Work out the finished part from the listing and answer in its coordinate system (mm). A direction names the side the tool comes from. Coordinates: 2 decimals unless noted, no trailing zeros. Order: outer loops, then holes, each group sorted by start corner. A loop starts at its lowest first (then second) coordinate and runs counter-clockwise, first axis right, second up. Notation, with made-up numbers: (15.5, 33) -> (46.5, 33) arc R14 cw to (46.5, 50) -> close; hole circle Ø11 at (72, 55). An arc over 180 degrees is marked (long way). Use one line per item in the form item = value.
from build123d import *

# Parameters (mm, degrees)
SKETCH1_W                      = 119.888
SKETCH1_H                      = 182.88
BOSS_EXTRUDE1_DEPTH            = 9.525
F_1_4_20_TAPPED_HOLE1_D        = 5.1054
CUT_EXTRUDE1_DEPTH             = 1.9685
CUT_EXTRUDE2_DEPTH             = 1.9685
F_6_32_TAPPED_HOLE1_AT_2_COUNT = 2
F_6_32_TAPPED_HOLE1_AT_2_PITCH = 93.98
F_6_32_TAPPED_HOLE1_AT_3_COUNT = 2
F_6_32_TAPPED_HOLE1_AT_3_PITCH = 82.55
F_6_32_TAPPED_HOLE1_AT_4_COUNT = 2
F_6_32_TAPPED_HOLE1_AT_4_PITCH = 11.43


with BuildPart() as part:
    # Sketch1 → Boss-Extrude1 (new body)
    with BuildSketch(Plane(origin=(0, 0, 0), x_dir=(1, 0, 0), z_dir=(0, 1, 0))):
        Rectangle(SKETCH1_W, SKETCH1_H)
        with BuildLine():
            Line((-29.26715, 79.502), (29.26715, 79.502))
            ThreePointArc((29.26715, 79.502), (29.828416008, 79.734483992), (30.0609, 80.29575))
            Line((30.0609, 80.29575), (30.0609, 85.56625))
            ThreePointArc((30.0609, 85.56625), (29.828416008, 86.127516008), (29.26715, 86.36))
            Line((29.26715, 86.36), (-29.26715, 86.36))
            ThreePointArc((-29.26715, 86.36), (-29.828416008, 86.127516008), (-30.0609, 85.56625))
            Line((-30.0609, 85.56625), (-30.0609, 80.29575))
            ThreePointArc((-30.0609, 80.29575), (-29.828416008, 79.734483992), (-29.26715, 79.502))
        make_face(mode=Mode.SUBTRACT)
        with BuildLine():
            Line((-29.26715, 64.6811), (29.26715, 64.6811))
            ThreePointArc((29.26715, 64.6811), (29.828416008, 64.913583992), (30.0609, 65.47485))
            Line((30.0609, 65.47485), (30.0609, 70.74535))
            ThreePointArc((30.0609, 70.74535), (29.828416008, 71.306616008), (29.26715, 71.5391))
            Line((29.26715, 71.5391), (-29.26715, 71.5391))
            ThreePointArc((-29.26715, 71.5391), (-29.828416008, 71.306616008), (-30.0609, 70.74535))
            Line((-30.0609, 70.74535), (-30.0609, 65.47485))
            ThreePointArc((-30.0609, 65.47485), (-29.828416008, 64.913583992), (-29.26715, 64.6811))
        make_face(mode=Mode.SUBTRACT)
        with BuildLine():
            Line((-52.54625, 19.1262), (-47.11065, 19.1262))
            ThreePointArc((-47.11065, 19.1262), (-46.549383992, 19.358683992), (-46.3169, 19.91995))
            Line((-46.3169, 19.91995), (-46.3169, 57.95645))
            ThreePointArc((-46.3169, 57.95645), (-46.549383992, 58.517716008), (-47.11065, 58.7502))
            Line((-47.11065, 58.7502), (-52.54625, 58.7502))
            ThreePointArc((-52.54625, 58.7502), (-53.107516008, 58.517716008), (-53.34, 57.95645))
            Line((-53.34, 57.95645), (-53.34, 19.91995))
            ThreePointArc((-53.34, 19.91995), (-53.107516008, 19.358683992), (-52.54625, 19.1262))
        make_face(mode=Mode.SUBTRACT)
        with BuildLine():
            Line((46.3169, 19.91995), (46.3169, 57.95645))
            ThreePointArc((46.3169, 57.95645), (46.549383992, 58.517716008), (47.11065, 58.7502))
            Line((47.11065, 58.7502), (52.54625, 58.7502))
            ThreePointArc((52.54625, 58.7502), (53.107516008, 58.517716008), (53.34, 57.95645))
            Line((53.34, 57.95645), (53.34, 19.91995))
            ThreePointArc((53.34, 19.91995), (53.107516008, 19.358683992), (52.54625, 19.1262))
            Line((52.54625, 19.1262), (47.11065, 19.1262))
            ThreePointArc((47.11065, 19.1262), (46.549383992, 19.358683992), (46.3169, 19.91995))
        make_face(mode=Mode.SUBTRACT)
    extrude(amount=BOSS_EXTRUDE1_DEPTH)

    # 1/4-20 Tapped Hole1 (through all)
    with Locations(Plane(origin=(0, 9.525, 0), x_dir=(1, 0, 0), z_dir=(0, 1, 0))):
        with Locations((-49.82845, -85.09), (49.82845, -85.09)):
            Hole(F_1_4_20_TAPPED_HOLE1_D / 2)

    # Sketch4 → Cut-Extrude1 (cut)
    with BuildSketch(Plane(origin=(0, 9.525, 0), x_dir=(1, 0, 0), z_dir=(0, 1, 0))):
        with BuildLine():
            Line((-30.0482, -91.44), (-24.4602, -91.44))
            Line((-24.4602, -91.44), (-24.4602, 56.3372))
            ThreePointArc((-24.4602, 56.3372), (-27.2542, 59.1312), (-30.0482, 56.3372))
            Line((-30.0482, 56.3372), (-30.0482, -91.44))
        make_face()
        with BuildLine():
            Line((-2.794, 56.3372), (-2.794, -91.44))
            Line((-2.794, -91.44), (2.794, -91.44))
            Line((2.794, -91.44), (2.794, 56.3372))
            ThreePointArc((2.794, 56.3372), (0, 59.1312), (-2.794, 56.3372))
        make_face()
        with BuildLine():
            Line((30.0482, 56.3372), (30.0482, -91.44))
            Line((30.0482, -91.44), (24.4602, -91.44))
            Line((24.4602, -91.44), (24.4602, 56.3372))
            ThreePointArc((24.4602, 56.3372), (27.2542, 59.1312), (30.0482, 56.3372))
        make_face()
    extrude(amount=-CUT_EXTRUDE1_DEPTH, mode=Mode.SUBTRACT)

    # Sketch5 → Cut-Extrude2 (cut)
    with BuildSketch(Plane.XZ):
        with BuildLine():
            Line((-40.005, -73.10755), (40.005, -73.10755))
            ThreePointArc((40.005, -73.10755), (42.418, -75.52055), (40.005, -77.93355))
            Line((40.005, -77.93355), (-40.005, -77.93355))
            ThreePointArc((-40.005, -77.93355), (-42.418, -75.52055), (-40.005, -73.10755))
        make_face()
        with BuildLine():
            Line((-40.005, -58.28665), (40.005, -58.28665))
            ThreePointArc((40.005, -58.28665), (42.418, -60.69965), (40.005, -63.11265))
            Line((40.005, -63.11265), (-40.005, -63.11265))
            ThreePointArc((-40.005, -63.11265), (-42.418, -60.69965), (-40.005, -58.28665))
        make_face()
    extrude(amount=-CUT_EXTRUDE2_DEPTH, mode=Mode.SUBTRACT)

    # Sketch7 → #6-32 Tapped Hole1 (revolve, cut)
    with BuildSketch(Plane(origin=(-59.944, 4.7625, 27.94), x_dir=(0, 0, 1), z_dir=(0, 1, 0))):
        Polygon((0, 0), (0, 13.51269403), (1.35255, 12.7), (1.35255, 0), align=None)
    f_6_32_tapped_hole1 = revolve(axis=Axis((-66.294, 4.7625, 27.94), (1, 0, 0)), mode=Mode.SUBTRACT)

    # #6-32 Tapped Hole1 at 2: #6-32 Tapped Hole1 ×2
    with Locations(*[(0, 0, -i * F_6_32_TAPPED_HOLE1_AT_2_PITCH) for i in range(1, F_6_32_TAPPED_HOLE1_AT_2_COUNT)]):
        add(f_6_32_tapped_hole1, mode=Mode.SUBTRACT)

    # #6-32 Tapped Hole1 at 3: #6-32 Tapped Hole1 ×2
    with Locations(*[(0, 0, -i * F_6_32_TAPPED_HOLE1_AT_3_PITCH) for i in range(1, F_6_32_TAPPED_HOLE1_AT_3_COUNT)]):
        add(f_6_32_tapped_hole1, mode=Mode.SUBTRACT)

    # #6-32 Tapped Hole1 at 4: #6-32 Tapped Hole1 ×2
    with Locations(*[(0, 0, -i * F_6_32_TAPPED_HOLE1_AT_4_PITCH) for i in range(1, F_6_32_TAPPED_HOLE1_AT_4_COUNT)]):
        add(f_6_32_tapped_hole1, mode=Mode.SUBTRACT)

    # Mirror1: #6-32 Tapped Hole1 across plane
    add(f_6_32_tapped_hole1.mirror(Plane(origin=(0, 0, 0), x_dir=(0, 0, 1), z_dir=(1, 0, 0))), mode=Mode.SUBTRACT)

    # Mirror1 copy 1 sketch → Mirror1 copy 1 (revolve, cut)
    with BuildSketch(Plane(origin=(59.944, 4.7625, -66.04), x_dir=(0, 0, 1), z_dir=(0, 1, 0))):
        Polygon((0, 0), (0, -13.51269403), (1.35255, -12.7), (1.35255, 0), align=None)
    revolve(axis=Axis((66.294, 4.7625, -66.04), (1, 0, 0)), mode=Mode.SUBTRACT)

    # Mirror1 copy 2 sketch → Mirror1 copy 2 (revolve, cut)
    with BuildSketch(Plane(origin=(59.944, 4.7625, -54.61), x_dir=(0, 0, 1), z_dir=(0, 1, 0))):
        Polygon((0, 0), (0, -13.51269403), (1.35255, -12.7), (1.35255, 0), align=None)
    revolve(axis=Axis((66.294, 4.7625, -54.61), (1, 0, 0)), mode=Mode.SUBTRACT)

    # Mirror1 copy 3 sketch → Mirror1 copy 3 (revolve, cut)
    with BuildSketch(Plane(origin=(59.944, 4.7625, 16.51), x_dir=(0, 0, 1), z_dir=(0, 1, 0))):
        Polygon((0, 0), (0, -13.51269403), (1.35255, -12.7), (1.35255, 0), align=None)
    revolve(axis=Axis((66.294, 4.7625, 16.51), (1, 0, 0)), mode=Mode.SUBTRACT)


solid = part.part
(1) Which of the six approach directions +Z, -Z, +X, -X, +Y, -Y give full straight-line access (tool end or side, diameter ignored) to faces 1 (the flat face through (-27, 7.557, 15)), 2 (the flat face through (-1, 5, -91.44)), 3 (the flat face through (-46.317, 5, -39))?
Data:
face_1 = +Z, +Y
face_2 = -Z, +X, -X, +Y, -Y
face_3 = +Y, -Y
(2) This flat-tipped pin is pushed along its axis until it touches: P1, Ø2, axis at y = 4.76, z = 16.51, coming from the +X side. Where does it stop, or does it pass through?
Data:
P1 = 47.03
(3) Straight lines are drawn through the part: line 1 along Z through (x, y) = (5, 9.25); line 2 along X through (y, z) = (8.25, 9); line 3 along Z through (x, y) = (-8.5, 1.5). For each, find the intervals that lie inside material, in ascending order.
Data:
line_1 = -91.44 to -86.36, -79.5 to -71.54, -64.68 to 91.44
line_2 = -59.94 to -30.05, -24.46 to -2.79, 2.79 to 24.46, 30.05 to 59.94
line_3 = -91.44 to -86.36, -79.5 to -77.93, -73.11 to -71.54, -64.68 to -63.11, -58.29 to 91.44
(4) The mould has two halves that part along Z. Classify faces 4 (the flat face through (-1, 0, 19)), 5 (the flat face through (0, 5, -71.539)), 6 (the flat face through (-1, 5, 91.44)): released by +Z, released by -Z, zero draft, split by the parting line, or undercut.
Data:
face_4 = zero draft
face_5 = undercut
face_6 = released by +Z
(5) Section B-B on z = 85.09 is taken. Write down the section's boundary in (x, y) (1 decimal), plus the area to 3 significant figures.
Data:
outline = (-59.9, 0) -> (-52.4, 0) -> (-52.4, 9.5) -> (-59.9, 9.5) -> close; (-47.3, 0) -> (47.3, 0) -> (47.3, 9.5) -> (30, 9.5) -> (30, 7.6) -> (24.5, 7.6) -> (24.5, 9.5) -> (2.8, 9.5) -> (2.8, 7.6) -> (-2.8, 7.6) -> (-2.8, 9.5) -> (-24.5, 9.5) -> (-24.5, 7.6) -> (-30, 7.6) -> (-30, 9.5) -> (-47.3, 9.5) -> close; (52.4, 0) -> (59.9, 0) -> (59.9, 9.5) -> (52.4, 9.5) -> close
area = 1,010 mm²
(6) Section D-D on x = 0 is taken. Write down the section's boundary in (y, z) (1 decimal).
Data:
outline = (0, -91.4) -> (9.5, -91.4) -> (9.5, -86.4) -> (0, -86.4) -> close; (0, -79.5) -> (9.5, -79.5) -> (9.5, -71.5) -> (0, -71.5) -> (0, -73.1) -> (2, -73.1) -> (2, -77.9) -> (0, -77.9) -> close; (0, -64.7) -> (9.5, -64.7) -> (9.5, -59.1) -> (7.6, -59.1) -> (7.6, 91.4) -> (0, 91.4) -> (0, -58.3) -> (2, -58.3) -> (2, -63.1) -> (0, -63.1) -> close
(7) Section C-C on z = 49 is taken. Write down the section's boundary in (x, y) (1 decimal), plus the area to 3 significant figures.
Data:
outline = (-59.9, 0) -> (59.9, 0) -> (59.9, 9.5) -> (30, 9.5) -> (30, 7.6) -> (24.5, 7.6) -> (24.5, 9.5) -> (2.8, 9.5) -> (2.8, 7.6) -> (-2.8, 7.6) -> (-2.8, 9.5) -> (-24.5, 9.5) -> (-24.5, 7.6) -> (-30, 7.6) -> (-30, 9.5) -> (-59.9, 9.5) -> close
area = 1,110 mm²
(8) Section A-A on x = 17 is taken. Write down the section's boundary in (y, z) (1 decimal).
Data:
outline = (0, -91.4) -> (9.5, -91.4) -> (9.5, -86.4) -> (0, -86.4) -> close; (0, -79.5) -> (9.5, -79.5) -> (9.5, -71.5) -> (0, -71.5) -> (0, -73.1) -> (2, -73.1) -> (2, -77.9) -> (0, -77.9) -> close; (0, -64.7) -> (9.5, -64.7) -> (9.5, 91.4) -> (0, 91.4) -> (0, -58.3) -> (2, -58.3) -> (2, -63.1) -> (0, -63.1) -> close
